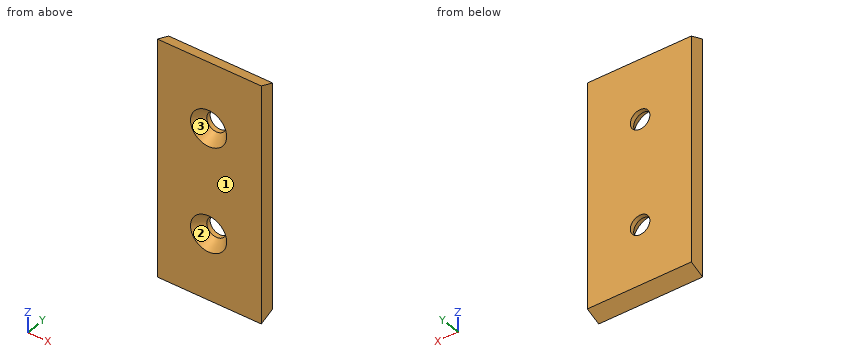
```python
from build123d import *

# Parameters (mm, degrees)
SKETCH_1_W                          = 69
SKETCH_1_H                          = 158
EXTRUDE_1_DEPTH                     = 10
CUT_EXTRUDE_2_REACH                 = 88.783
SKETCH_4_R                          = 6.5
CHAMFER_1_SIZE                      = 5.5
CHAMFER_1_SIZE2                     = 7
PATTERN_LINEAR_2_COUNT              = 2
PATTERN_LINEAR_2_PITCH              = 70
CHAMFER_1_OF_PATTERN_LINEAR_2_SIZE2 = 7
CHAMFER_1_OF_PATTERN_LINEAR_2_SIZE  = 5.5
CUT_EXTRUDE_3_REACH                 = 107.366


with BuildPart() as part:
    # 草图1 → 凸台-拉伸1 (new body)
    with BuildSketch(Plane(origin=(0, 0, 0), x_dir=(1, 0, 0), z_dir=(0, 1, 0))):
        Rectangle(SKETCH_1_W, SKETCH_1_H)
    extrude(amount=EXTRUDE_1_DEPTH)

    # 草图4 → 切除-拉伸2 (cut, up to next)
    with BuildSketch(Plane.XZ, mode=Mode.PRIVATE) as cut_extrude_2_sk1:
        with Locations(Location((-0.5, 35, 0), (0, 0, 270))):
            Circle(SKETCH_4_R)
    cut_extrude_2_tool1 = extrude(cut_extrude_2_sk1.sketch, amount=-CUT_EXTRUDE_2_REACH, mode=Mode.PRIVATE) & part.part
    cut_extrude_2 = cut_extrude_2_tool1.solids().sort_by_distance((-0.5, 0, 35))[0]
    add(cut_extrude_2, mode=Mode.SUBTRACT)

    # 倒角1
    chamfer_1_edges = [part.edges().sort_by_distance(p)[0] for p in [
        (-0.5, 0, 41.5),
    ]]
    chamfer_1_side = [part.faces().sort_by_distance(p)[0] for p in [
        (0.006162549, 0, -0.431378462),
    ]]
    chamfer(chamfer_1_edges, length=CHAMFER_1_SIZE, length2=CHAMFER_1_SIZE2, reference=chamfer_1_side[0])

    # 阵列(线性)2: 切除-拉伸2 ×2
    with Locations(*[(0, 0, -i * PATTERN_LINEAR_2_PITCH) for i in range(1, PATTERN_LINEAR_2_COUNT)]):
        add(cut_extrude_2, mode=Mode.SUBTRACT)

    # 倒角1 of 阵列(线性)2
    chamfer_1_of_pattern_linear_2_edges = [part.edges().sort_by_distance(p)[0] for p in [
        (-0.5, 0, -28.5),
    ]]
    chamfer(chamfer_1_of_pattern_linear_2_edges, length=CHAMFER_1_OF_PATTERN_LINEAR_2_SIZE, length2=CHAMFER_1_OF_PATTERN_LINEAR_2_SIZE2)

    # 草图6 → 切除-拉伸3 (cut, up to next)
    with BuildSketch(Plane(origin=(34.5, 0, 0), x_dir=(0, 0, -1), z_dir=(1, 0, 0)), mode=Mode.PRIVATE) as cut_extrude_3_sk1:
        Polygon((-79, 0), (-75.000285359, 10), (-79, 10), align=None)
    cut_extrude_3_tool1 = extrude(cut_extrude_3_sk1.sketch, amount=-CUT_EXTRUDE_3_REACH, mode=Mode.PRIVATE) & part.part
    # 草图6 → 切除-拉伸3 (cut, up to next)
    with BuildSketch(Plane(origin=(34.5, 0, 0), x_dir=(0, 0, -1), z_dir=(1, 0, 0)), mode=Mode.PRIVATE) as cut_extrude_3_sk2:
        Polygon((79, 10), (79, 0), (75.000285359, 10), align=None)
    cut_extrude_3_tool2 = extrude(cut_extrude_3_sk2.sketch, amount=-CUT_EXTRUDE_3_REACH, mode=Mode.PRIVATE) & part.part
    add(cut_extrude_3_tool1.solids().sort_by_distance((34.5, 6.666667, 77.666762))[0], mode=Mode.SUBTRACT)
    add(cut_extrude_3_tool2.solids().sort_by_distance((34.5, 6.666667, -77.666762))[0], mode=Mode.SUBTRACT)


solid = part.part
```
CAD build for the part. Positions are in the model's coordinates, mm. Face numbers are marked on the shaded views. Give positions to 0.01 mm unless a question says otherwise; leave off trailing zeros. Write each loop counter-clockwise with the first axis right and the second up, starting at its lowest first coordinate (ties: lowest second). Pieces come first, ordered by that corner, then holes. Notation, with made-up numbers: M 44.5,44 L 70.5,44 A15 cw 70.5,55 Z; hole C 41.25,-29 d1. An arc over 180 degrees is marked long. Return JSON: item names as keys, results as strings. Group by question number.
(1) Mould opens along X. For the marked faces 1, 2 and 3 say: pulls with the +X half, pulls with the -X half, needs draft (parallel to the pull), parting line crosses it, or undercut.
(2) Band-saw the part on B-B (z = -35). Give the cut face in (x, y), and give its area (4 significant figures).
(3) Band-saw the part on C-C (y = 2.5). Give the cut face in (x, z).
(4) Band-saw the part on A-A (x = -0.5). Give the cut face in (y, z), and give its area (3 significant figures).
(5) Drill centre lines: L1, parallel to X at y = 8.8, z = 35; L2, parallel to Z at x = 3.5, y = 8; L3, parallel to Z at x = 1, y = 8.75. Where is each one in solid material? Low to high. Write a range as [from, to].
(6) Band-saw the part on D-D (x = 24.5). Give the cut face in (y, z).
(7) Flat gauge pins, fed straight in: pin 1 Ø6 at (x, z) = (-10.5, -30.5) entering from -Y; pin 2 Ø3 at (x, y) = (-9.5, 9) entering from -Z. Where does each tip first touch, or does it go through?
Entries:
{
 "1": {"face 1": "needs draft", "face 2": "undercut", "face 3": "undercut"},
 "2": {"outline": "M -34.5,0 L -12.5,0 L -7,7 L -7,10 L -34.5,10 Z; M 6,7 L 11.5,0 L 34.5,0 L 34.5,10 L 6,10 Z", "area": "521.5 mm^2"},
 "3": {"outline": "M -34.5,-78 L 34.5,-78 L 34.5,78 L -34.5,78 Z; hole C -0.5,-35 d20.07; hole C -0.5,35 d20.07"},
 "4": {"outline": "M 0,-79 L 10,-75 L 10,-41.5 L 7,-41.5 L 0,-47 Z; M 0,-23 L 7,-28.5 L 10,-28.5 L 10,28.5 L 7,28.5 L 0,23 Z; M 0,47 L 7,41.5 L 10,41.5 L 10,75 L 0,79 Z", "area": "1,200 mm^2"},
 "5": {"L1": "x = [-34.5, -7], [6, 34.5]", "L2": "z = [-75.8, -40.12], [-29.88, 29.88], [40.12, 75.8]", "L3": "z = [-75.5, -41.32], [-28.68, 28.68], [41.32, 75.5]"},
 "6": {"outline": "M 0,-79 L 10,-75 L 10,75 L 0,79 Z"},
 "7": {"pin 1": "stops at y = 0", "pin 2": "stops at z = -76"}
}
